from build123d import *

# Parameters (mm, degrees)
CSK_FOR_M10_COUNTERSUNK_FLAT_HEAD_SCREW1_D           = 11
CSK_FOR_M10_COUNTERSUNK_FLAT_HEAD_SCREW1_DEPTH       = 10.695266595
CSK_FOR_M10_COUNTERSUNK_FLAT_HEAD_SCREW1_CSINK_D     = 14
CSK_FOR_M10_COUNTERSUNK_FLAT_HEAD_SCREW1_CSINK_ANGLE = 90
CSK_FOR_M10_COUNTERSUNK_FLAT_HEAD_SCREW1_TIP         = 3.304733405
CSK_FOR_M10_COUNTERSUNK_FLAT_HEAD_SCREW2_D           = 11
CSK_FOR_M10_COUNTERSUNK_FLAT_HEAD_SCREW2_DEPTH       = 10.695266595
CSK_FOR_M10_COUNTERSUNK_FLAT_HEAD_SCREW2_CSINK_D     = 14
CSK_FOR_M10_COUNTERSUNK_FLAT_HEAD_SCREW2_CSINK_ANGLE = 90
CSK_FOR_M10_COUNTERSUNK_FLAT_HEAD_SCREW2_TIP         = 3.304733405


with BuildPart() as part:
    # Sketch1 → Revolve1 (revolve)
    with BuildSketch(Plane.XY):
        Polygon((0, 0), (0, 12.2), (2.5, 14.7), (17, 14.7), (17, 37.5), (109.5, 37.5), (109.5, 35), (141.5, 35), (141.5, 33), (196, 33), (196, 27.5), (286, 27.5), (286, 24), (308, 24), (308, 20), (321.5, 20), (323, 18.5), (323, 0), align=None)
    revolve(axis=Axis((0, 0, 0), (1, 0, 0)))

    # CSK for M10 Countersunk Flat Head Screw1
    with Locations(Plane.ZY):
        with Locations((0, 0)):
            CounterSinkHole(CSK_FOR_M10_COUNTERSUNK_FLAT_HEAD_SCREW1_D / 2, CSK_FOR_M10_COUNTERSUNK_FLAT_HEAD_SCREW1_CSINK_D / 2, depth=CSK_FOR_M10_COUNTERSUNK_FLAT_HEAD_SCREW1_DEPTH, counter_sink_angle=CSK_FOR_M10_COUNTERSUNK_FLAT_HEAD_SCREW1_CSINK_ANGLE)
            with Locations((0, 0, -(CSK_FOR_M10_COUNTERSUNK_FLAT_HEAD_SCREW1_DEPTH + CSK_FOR_M10_COUNTERSUNK_FLAT_HEAD_SCREW1_TIP / 2))):  # 118° drill point
                Cone(0, CSK_FOR_M10_COUNTERSUNK_FLAT_HEAD_SCREW1_D / 2, CSK_FOR_M10_COUNTERSUNK_FLAT_HEAD_SCREW1_TIP, mode=Mode.SUBTRACT)

    # CSK for M10 Countersunk Flat Head Screw2
    with Locations(Plane(origin=(323, 0, 0), x_dir=(0, 0, -1), z_dir=(1, 0, 0))):
        with Locations((0, 0)):
            CounterSinkHole(CSK_FOR_M10_COUNTERSUNK_FLAT_HEAD_SCREW2_D / 2, CSK_FOR_M10_COUNTERSUNK_FLAT_HEAD_SCREW2_CSINK_D / 2, depth=CSK_FOR_M10_COUNTERSUNK_FLAT_HEAD_SCREW2_DEPTH, counter_sink_angle=CSK_FOR_M10_COUNTERSUNK_FLAT_HEAD_SCREW2_CSINK_ANGLE)
            with Locations((0, 0, -(CSK_FOR_M10_COUNTERSUNK_FLAT_HEAD_SCREW2_DEPTH + CSK_FOR_M10_COUNTERSUNK_FLAT_HEAD_SCREW2_TIP / 2))):  # 118° drill point
                Cone(0, CSK_FOR_M10_COUNTERSUNK_FLAT_HEAD_SCREW2_D / 2, CSK_FOR_M10_COUNTERSUNK_FLAT_HEAD_SCREW2_TIP, mode=Mode.SUBTRACT)


solid = part.part
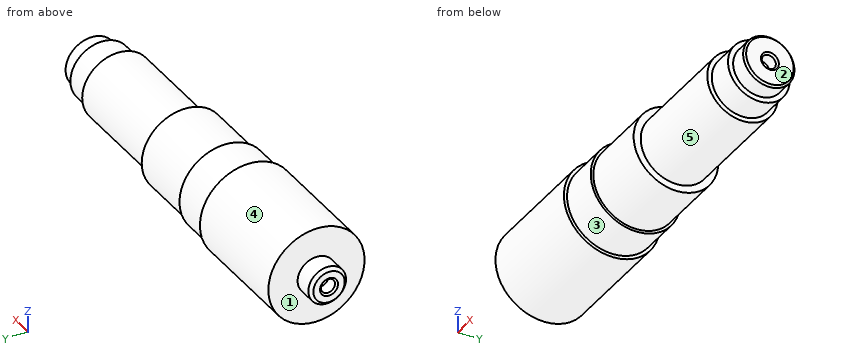
Geometry check sheet. Reference: the model listing, model coordinates, mm. Face numbers are marked on the shaded views. A direction names the side the tool comes from. Give positions to 0.01 mm unless a question says otherwise; leave off trailing zeros. Order: outer loops, then holes, each group sorted by start corner. A loop starts at its lowest first (then second) coordinate and runs counter-clockwise, first axis right, second up. Notation, with made-up numbers: (-2, -1) - (28, -1) arc R32 ccw to (28, 27) - close; hole circle Ø7 at (83, 23). An arc over 180 degrees is marked (long way). Use one line per item in the form item = value.
1) Draft check along X on the marked faces 1, 2 and 3. Enter one of: released by +X, released by -X, zero draft, split by the parting line, or undercut.
Working result:
face_1 = released by -X
face_2 = released by +X
face_3 = zero draft
2) Sectioned sample at B-B (x = 159). Record the boundary of the cut face in (y, z).
Working result:
outline = circle Ø66 at (0, 0)
3) Depth check by flat-ended pin: pin 1 Ø5 at (y, z) = (-20.5, -10) entering from +X; pin 2 Ø6 at (x, z) = (188, 26) entering from -Y; pin 3 Ø1 at (x, y) = (274.5, -9) entering from -Z. Enter the tip coordinate at first touch or a pass-through.
Working result:
pin_1 = 308
pin_2 = -23.66
pin_3 = -26.15
4) Sectioned sample at A-A (x = 85). Record the boundary of the cut face in (y, z).
Working result:
outline = circle Ø75 at (0, 0)
5) Material ranges on probe 1 along Z at (x, y) = (317, 0); probe 2 along Z at (x, y) = (8.25, 0); probe 3 along X at (y, z) = (14, -23), recorded low to high. Write a range as from..to.
Working result:
probe_1 = -20..-5.5, 5.5..20
probe_2 = -14.7..-5.5, 5.5..14.7
probe_3 = 17..286
6) Access from +Z, -Z, +X, -X, +Y, -Y to the whole of each face (thin tool, end or side, straight path). Record for the marked faces 4 and 5.
Working result:
face_4 = +X, -X
face_5 = +X
